Check sheet for the modelled part. Datum: model origin and axes. Units: mm. Face numbers are marked on the shaded views. A direction names the side the tool comes from. Round coordinates to 2 decimals unless told otherwise and drop trailing zeros. Loops run counter-clockwise (first coordinate to the right, second up) from the corner with the lowest first, then second, coordinate; pieces in that order, holes last. Notation, with made-up numbers: (17, 82.5) -> (37, 82.5) arc R21 ccw to (37, 117.5) -> close; hole circle Ø9 at (-8, -19). An arc over 180 degrees is marked (long way). One line per question, with ' | ' between items.
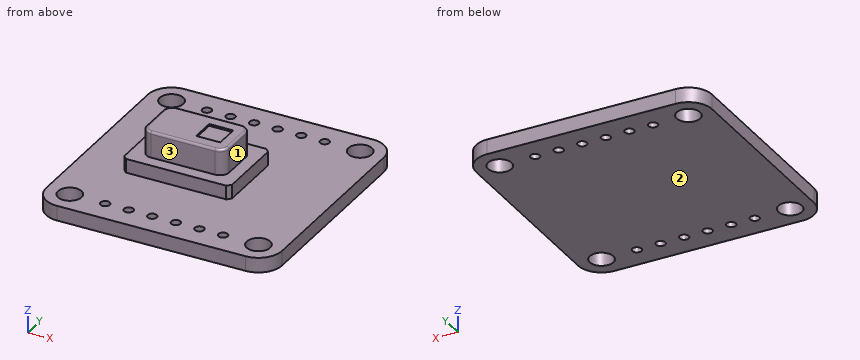
Autodesk Fusion 360 part; units mm, degrees
sketch "AMG8833_REV-B" plane through (0, 0, 0) normal (0, 0, 1) x (1, 0, 0)
  arc A0 (2.54, 25.4) -> (0, 22.86) centre (2.54, 22.86) ccw
  line L0 (2.54, 25.4) -> (22.86, 25.4)
  line L1 (22.86, 0) -> (2.54, 0)
  arc A1 (0, 2.54) -> (2.54, 0) centre (2.54, 2.54) ccw
  line L2 (0, 2.54) -> (0, 22.86)
  arc A2 (22.86, 0) -> (25.4, 2.54) centre (22.86, 2.54) ccw
  arc A3 (25.4, 22.86) -> (22.86, 25.4) centre (22.86, 22.86) ccw
  line L3 (25.4, 22.86) -> (25.4, 2.54)
  circle A4 centre (2.54, 22.86) radius 1.758
  circle A5 centre (8.89, 2.54) radius 0.889
  circle A6 centre (2.54, 22.86) radius 1.758
  circle A7 centre (11.43, 2.54) radius 0.889
  circle A8 centre (22.86, 22.86) radius 1.758
  circle A9 centre (22.86, 2.54) radius 1.758
  circle A10 centre (6.35, 2.54) radius 0.889
  circle A11 centre (22.86, 2.54) radius 1.758
  circle A12 centre (11.43, 2.54) radius 0.889
  circle A13 centre (16.51, 22.86) radius 0.889
  circle A14 centre (13.97, 22.86) radius 0.889
  circle A15 centre (6.35, 22.86) radius 0.889
  circle A16 centre (6.35, 22.86) radius 0.889
  circle A17 centre (2.54, 2.54) radius 1.758
  circle A18 centre (19.05, 22.86) radius 0.889
  circle A19 centre (8.89, 22.86) radius 0.889
  circle A20 centre (11.43, 22.86) radius 0.889
  circle A21 centre (11.43, 22.86) radius 0.889
  circle A22 centre (13.97, 2.54) radius 0.889
  circle A23 centre (16.51, 2.54) radius 0.889
  circle A24 centre (16.51, 2.54) radius 0.889
  circle A25 centre (19.05, 22.86) radius 0.889
  circle A26 centre (16.51, 22.86) radius 0.889
  circle A27 centre (13.97, 22.86) radius 0.889
  circle A28 centre (8.89, 22.86) radius 0.889
  circle A29 centre (6.35, 2.54) radius 0.889
  circle A30 centre (19.05, 2.54) radius 0.889
  circle A31 centre (8.89, 2.54) radius 0.889
  circle A32 centre (13.97, 2.54) radius 0.889
  circle A33 centre (22.86, 22.86) radius 1.758
  circle A34 centre (2.54, 2.54) radius 1.758
  circle A35 centre (19.05, 2.54) radius 0.889
extrude "Extrude2" add sketch "AMG8833_REV-B" along normal blind 1.6
sketch "holes" plane through (0, 0, 1.6) normal (0, 0, 1) x (-1, 0, 0)
  circle A0 centre (-19.05, -2.54) radius 0.889
  circle A1 centre (-6.35, -22.86) radius 0.889
  circle A2 centre (-2.54, -2.54) radius 1.758
  circle A3 centre (-13.97, -22.86) radius 0.889
  circle A4 centre (-19.05, -22.86) radius 0.889
  circle A5 centre (-22.86, -2.54) radius 1.758
  circle A6 centre (-22.86, -22.86) radius 1.758
  circle A7 centre (-6.35, -2.54) radius 0.889
  circle A8 centre (-16.51, -2.54) radius 0.889
  circle A9 centre (-2.54, -22.86) radius 1.758
  circle A10 centre (-13.97, -2.54) radius 0.889
  circle A11 centre (-8.89, -2.54) radius 0.889
  circle A12 centre (-8.89, -22.86) radius 0.889
  circle A13 centre (-11.43, -22.86) radius 0.889
  circle A14 centre (-11.43, -2.54) radius 0.889
  circle A15 centre (-16.51, -22.86) radius 0.889
  arc A16 (-2.54, -25.4) -> (0, -22.86) centre (-2.54, -22.86) ccw
  line L0 (0, -22.86) -> (0, -2.54)
  arc A17 (0, -2.54) -> (-2.54, 0) centre (-2.54, -2.54) ccw
  line L1 (-2.54, 0) -> (-22.86, 0)
  arc A18 (-22.86, 0) -> (-25.4, -2.54) centre (-22.86, -2.54) ccw
  line L2 (-25.4, -2.54) -> (-25.4, -22.86)
  arc A19 (-25.4, -22.86) -> (-22.86, -25.4) centre (-22.86, -22.86) ccw
  line L3 (-22.86, -25.4) -> (-2.54, -25.4)
  circle A20 centre (-22.86, -22.86) radius 1.27
  circle A21 centre (-2.54, -22.86) radius 1.27
  circle A22 centre (-2.54, -2.54) radius 1.27
  circle A23 centre (-22.86, -2.54) radius 1.27
  circle A24 centre (-19.05, -2.54) radius 0.5
  circle A25 centre (-16.51, -2.54) radius 0.5
  circle A26 centre (-13.97, -2.54) radius 0.5
  circle A27 centre (-11.43, -2.54) radius 0.5
  circle A28 centre (-8.89, -2.54) radius 0.5
  circle A29 centre (-6.35, -2.54) radius 0.5
  circle A30 centre (-19.05, -22.86) radius 0.5
  circle A31 centre (-16.51, -22.86) radius 0.5
  circle A32 centre (-13.97, -22.86) radius 0.5
  circle A33 centre (-11.43, -22.86) radius 0.5
  circle A34 centre (-8.89, -22.86) radius 0.5
  circle A35 centre (-6.35, -22.86) radius 0.5
  dimension "d5" = 2.54
  dimension "d6" = 2.54
  dimension "d7" = 2.54
  dimension "d8" = 2.54
  dimension "d9" = 1
  dimension "d15" = 2.54
  dimension "d16" = 0
  dimension "d17" = 1
  dimension "d20" = 2.54
  dimension "d21" = 0
extrude "Extrude3" add sketch "holes" against normal blind 1.6 contours A0 | A1 | A2 | A3 | A4 | A5 | A6 | A7 | A8 | A9 | A10 | A11 | A12 | A13 | A14 | A15
sketch "lens base" plane through (0, 0, 1.6) normal (0, 0, 1) x (-1, 0, 0)
  circle A0 centre (-22.86, -2.54) radius 1.27
  circle A1 centre (-11.43, -2.54) radius 0.5
  circle A2 centre (-22.86, -22.86) radius 1.27
  circle A3 centre (-11.43, -22.86) radius 0.5
  circle A4 centre (-2.54, -22.86) radius 1.27
  circle A5 centre (-13.97, -22.86) radius 0.5
  circle A6 centre (-2.54, -2.54) radius 1.27
  circle A7 centre (-13.97, -2.54) radius 0.5
  circle A8 centre (-19.05, -2.54) radius 0.5
  circle A9 centre (-8.89, -2.54) radius 0.5
  circle A10 centre (-19.05, -22.86) radius 0.5
  circle A11 centre (-8.89, -22.86) radius 0.5
  circle A12 centre (-6.35, -22.86) radius 0.5
  circle A13 centre (-16.51, -22.86) radius 0.5
  circle A14 centre (-6.35, -2.54) radius 0.5
  circle A15 centre (-16.51, -2.54) radius 0.5
  arc A16 (-2.54, -25.4) -> (0, -22.86) centre (-2.54, -22.86) ccw
  line L0 (0, -22.86) -> (0, -2.54)
  arc A17 (0, -2.54) -> (-2.54, 0) centre (-2.54, -2.54) ccw
  line L1 (-2.54, 0) -> (-22.86, 0)
  arc A18 (-22.86, 0) -> (-25.4, -2.54) centre (-22.86, -2.54) ccw
  line L2 (-25.4, -2.54) -> (-25.4, -22.86)
  arc A19 (-25.4, -22.86) -> (-22.86, -25.4) centre (-22.86, -22.86) ccw
  line L3 (-22.86, -25.4) -> (-2.54, -25.4)
  line L4 (-4.868, -16.7) -> (-16.468, -16.7)
  line L5 (-16.468, -16.7) -> (-16.468, -8.7)
  line L6 (-16.468, -8.7) -> (-4.868, -8.7)
  line L7 (-4.868, -8.7) -> (-4.868, -16.7)
  line L8 (-10.668, -16.7) -> (-10.668, -8.7) construction
  line L9 (-16.468, -12.7) -> (-4.868, -12.7) construction
  dimension "d24" = 11.6
  dimension "d25" = 8
  dimension "d26" = 10.668
  dimension "d27" = 12.7
extrude "Extrude4" add sketch "lens base" along normal blind 1.5 contours L4 L5 L6 L7
sketch "lens" plane through (0, 0, 3.1) normal (0, 0, 1) x (-1, 0, 0)
  line L0 (-4.868, -8.7) -> (-16.468, -8.7)
  line L1 (-16.468, -8.7) -> (-16.468, -16.7)
  line L2 (-16.468, -16.7) -> (-4.868, -16.7)
  line L3 (-4.868, -16.7) -> (-4.868, -8.7)
  line L4 (-11.368, -14) -> (-13.968, -14)
  line L5 (-13.968, -14) -> (-13.968, -11.4)
  line L6 (-13.968, -11.4) -> (-11.368, -11.4)
  line L7 (-11.368, -11.4) -> (-11.368, -14)
  line L8 (-11.368, -12.7) -> (-13.968, -12.7) construction
  line L9 (-12.668, -14) -> (-12.668, -11.4) construction
  line L10 (-10.668, -16.7) -> (-10.668, -8.7) construction
  line L11 (-4.868, -12.7) -> (-16.468, -12.7) construction
  line L12 (-6.218, -15.35) -> (-15.118, -15.35)
  line L13 (-15.118, -15.35) -> (-15.118, -10.05)
  line L14 (-15.118, -10.05) -> (-6.218, -10.05)
  line L15 (-6.218, -10.05) -> (-6.218, -15.35)
  line L16 (-10.668, -15.35) -> (-10.668, -10.05) construction
  line L17 (-6.218, -12.7) -> (-15.118, -12.7) construction
  dimension "d30" = 2.6
  dimension "d31" = 2.6
  dimension "d32" = 2
  dimension "d33" = 8.9
  dimension "d34" = 5.3
extrude "Extrude5" add sketch "lens" along normal blind 2.8 contours L4 L5 L6 L7 | L12 L13 L14 L15
fillet "Fillet1" radius 1 4 edges at (6.218, 10.05, 4.5) (6.218, 15.35, 4.5) (15.118, 10.05, 4.5) (15.118, 15.35, 4.5)
fillet "Fillet2" radius 0.25 8 edges at (6.5109, 15.0571, 5.9) (6.218, 12.7, 5.9) (6.5109, 10.3429, 5.9) (10.668, 10.05, 5.9) (14.8251, 10.3429, 5.9) (15.118, 12.7, 5.9) (14.8251, 15.0571, 5.9) (10.668, 15.35, 5.9)
chamfer "Chamfer1" distance 0.4 angle 45 4 edges at (4.868, 16.7, 2.35) (4.868, 8.7, 2.35) (16.468, 16.7, 2.35) (16.468, 8.7, 2.35)
extrude "Extrude6" cut sketch "lens" against normal blind 0.2 from surface at 2.8 contours L4 L5 L6 L7
(1) Sectioned sample at B-B, the plane z = 0.5. Count the separate pieces of the cut face and the enclosed holes in it, and give its area (3 significant figures).
Answer:
separate pieces: 1 | enclosed holes: 16 | area: 610 mm2
(2) Set-up check for the marked faces 1, 2 and 3: record each of +Z, -Z, +X, -X, +Y, -Y from which the full face is reachable in a straight line by a thin tool's end or side.
Answer:
face 1: +Z, +X, +Y, -Y | face 2: -Z, +X, -X, +Y, -Y | face 3: +Z, +X, -X, -Y
(3) Scan lines: probe 1 along Y at (x, z) = (11.43, 0.4); probe 2 along Y at (x, z) = (8, 2.1); probe 3 along X at (y, z) = (22, 1). Record each from-to range of solid material in increasing order.
Answer:
probe 1: y = 0 to 2.04, 3.04 to 22.36, 23.36 to 25.4 | probe 2: y = 8.7 to 16.7 | probe 3: x = 0 to 1.61, 3.47 to 21.93, 23.79 to 25.4
(4) Sectioned sample at D-D, the plane x = 19.05. Record the cut outline in (y, z), and give its area (3 significant figures).
Answer:
outline: (0, 0) -> (2.04, 0) -> (2.04, 1.6) -> (0, 1.6) -> close; (3.04, 0) -> (22.36, 0) -> (22.36, 1.6) -> (3.04, 1.6) -> close; (23.36, 0) -> (25.4, 0) -> (25.4, 1.6) -> (23.36, 1.6) -> close | area: 37.4 mm2
(5) Sectioned sample at C-C, the plane z = 5.1. Record the cut outline in (x, y).
Answer:
outline: (6.22, 11.05) arc R1 ccw to (7.22, 10.05) -> (14.12, 10.05) arc R1 ccw to (15.12, 11.05) -> (15.12, 14.35) arc R1 ccw to (14.12, 15.35) -> (7.22, 15.35) arc R1 ccw to (6.22, 14.35) -> close
(6) Go/stop test with flat-tipped pins: pin 1 (3 mm diameter, centred on y = 12.5, z = 4.5, fed in from -X); pin 2 (5 mm diameter, centred on x = 17.5, y = 19, fed in from +Z); pin 3 (2 mm diameter, centred on x = 13.5, y = 16.5, fed in from +Z). Record where each tip stops, or that it passes through.
Answer:
pin 1: stops at x = 4.87 | pin 2: stops at z = 1.6 | pin 3: stops at z = 3.1
(7) Sectioned sample at A-A, the plane x = 8.89. Record the cut outline in (y, z).
Answer:
outline: (0, 0) -> (2.04, 0) -> (2.04, 1.6) -> (0, 1.6) -> close; (3.04, 0) -> (22.36, 0) -> (22.36, 1.6) -> (16.7, 1.6) -> (16.7, 3.1) -> (15.35, 3.1) -> (15.35, 5.65) arc R0.25 ccw to (15.1, 5.9) -> (10.3, 5.9) arc R0.25 ccw to (10.05, 5.65) -> (10.05, 3.1) -> (8.7, 3.1) -> (8.7, 1.6) -> (3.04, 1.6) -> close; (23.36, 0) -> (25.4, 0) -> (25.4, 1.6) -> (23.36, 1.6) -> close
